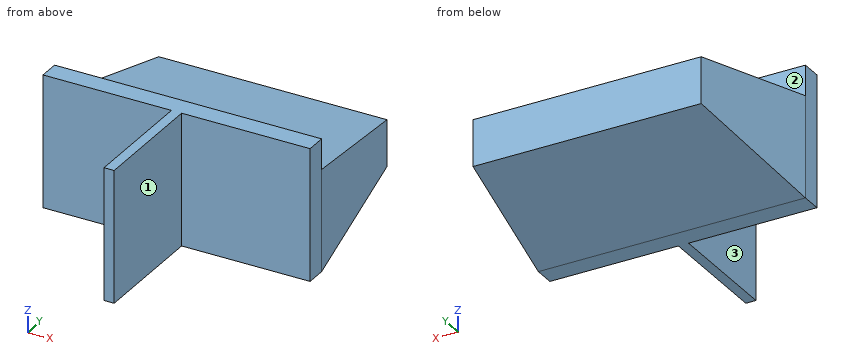
from build123d import *

# Parameters (mm, degrees)
SKETCH2_W           = 40.132
SKETCH2_H           = 19.812
BOSS_EXTRUDE1_DEPTH = 3.048
SKETCH3_W           = 40.132
SKETCH3_H           = 15.24
SKETCH4_W           = 34.29
SKETCH4_H           = 6.985
SKETCH5_W           = 1.524
SKETCH5_H           = 19.812
BOSS_EXTRUDE2_DEPTH = 17.78


with BuildPart() as part:
    # Sketch2 → Boss-Extrude1 (new body)
    with BuildSketch(Plane(origin=(0, 3.048, 0), x_dir=(1, 0, 0), z_dir=(0, 1, 0))):
        with Locations((20.066, 9.906)):
            Rectangle(SKETCH2_W, SKETCH2_H)
    extrude(amount=-BOSS_EXTRUDE1_DEPTH)

    # Sketch3 → Loft1 section 0
    with BuildSketch(Plane(origin=(0, 3.048, 0), x_dir=(1, 0, 0), z_dir=(0, 1, 0))):
        with Locations((20.066, 12.192)):
            Rectangle(SKETCH3_W, SKETCH3_H)
    # Sketch4 → Loft1 section 1
    with BuildSketch(Plane(origin=(0, 25.4, 0), x_dir=(1, 0, 0), z_dir=(0, 1, 0))):
        with Locations((20.066, 12.192)):
            Rectangle(SKETCH4_W, SKETCH4_H)
    loft()

    # Sketch5 → Boss-Extrude2 (add)
    with BuildSketch(Plane(origin=(0, 0, 0), x_dir=(1, 0, 0), z_dir=(0, 1, 0))):
        with Locations((20.066, 9.906)):
            Rectangle(SKETCH5_W, SKETCH5_H)
    extrude(amount=-BOSS_EXTRUDE2_DEPTH)


solid = part.part
Could you check a few things on this model? Use its own coordinates, in mm. Face numbers are marked on the shaded views. A direction names the side the tool comes from. Give positions to 0.01 mm unless a question says otherwise; leave off trailing zeros. Order: outer loops, then holes, each group sorted by start corner. A loop starts at its lowest first (then second) coordinate and runs counter-clockwise, first axis right, second up.
1. Suppose I cut it at A-A (z = -1.25). List the corners of the cut face in (x, y) for me.
2. Suppose I cut it at B-B (y = -5). List the corners of the cut face in (x, z) for me, plus the area to 3 significant figures.
3. I need wall thicknesses on L1, parallel to X at y = -16, z = -14.5; L2, parallel to Y at x = 25.5, z = -15.25; L3, parallel to Y at x = 25, z = -2.25. Which ranges of each line are inside material? Lowest first, please.
4. Will these pins go through, and if not, where does the flat tip stop? P1, Ø1.5, axis at x = 17, y = 4, coming from the -Z side; P2, Ø2, axis at x = 21, z = -9, coming from the -Y side; P3, Ø6, axis at x = 7.5, z = -9.5, coming from the -Y side; P4, Ø9, axis at y = -7, z = -9, coming from the -X side.
5. For the marked faces 1, 2 and 3, which set-ups out of +Z, -Z, +X, -X, +Y, -Y let a thin tool reach every point of the face, with its end or its side?
Solved:
1. outline: (0, 0) - (19.3, 0) - (19.3, -17.78) - (20.83, -17.78) - (20.83, 0) - (40.13, 0) - (40.13, 3.05) - (0, 3.05) - close
2. outline: (19.3, -19.81) - (20.83, -19.81) - (20.83, 0) - (19.3, 0) - close
2. area: 30.2 mm2
3. L1: x = 19.3 to 20.83
3. L2: y = 0 to 25.4
3. L3: y = 0 to 3.05
4. P1: stops at z = -19.77
4. P2: stops at y = -17.78
4. P3: stops at y = 0
4. P4: stops at x = 19.3
5. face 1: +Z, -Z, +X, -Y
5. face 2: +Z, +X, -X, +Y
5. face 3: +Z, -Z, -X, -Y
